Autodesk Fusion 360 part; units mm, degrees
sketch "Sketch1" plane through (0, 0, 0) normal (0, 0, 1) x (1, 0, 0)
  line L0 (-40, -75) -> (40, -75)
  line L1 (90, -25) -> (90, 25)
  line L2 (40, 75) -> (-40, 75)
  line L3 (-90, 25) -> (-90, -25)
  line L4 (-90, -75) -> (90, 75) construction
  line L5 (90, -75) -> (-90, 75) construction
  arc A0 (40, -75) -> (90, -25) centre (40, -25) ccw
  arc A1 (90, 25) -> (40, 75) centre (40, 25) ccw
  arc A2 (-90, -25) -> (-40, -75) centre (-40, -25) ccw
  arc A3 (-40, 75) -> (-90, 25) centre (-40, 25) ccw
extrude "Extrude1" add sketch "Sketch1" along normal blind 30
sketch "Sketch2" plane through (0, 0, 30) normal (0, 0, 1) x (-1, 0, 0)
  arc A0 (40, -75) -> (90, -25) centre (40, -25) ccw
  line L0 (90, -25) -> (90, 25)
  arc A1 (90, 25) -> (40, 75) centre (40, 25) ccw
  line L1 (40, 75) -> (-40, 75)
  arc A2 (-40, 75) -> (-90, 25) centre (-40, 25) ccw
  line L2 (-90, 25) -> (-90, -25)
  arc A3 (-90, -25) -> (-40, -75) centre (-40, -25) ccw
  line L3 (-40, -75) -> (40, -75)
  line L4 (35, 70) -> (-35, 70)
  line L5 (-85, 20) -> (-85, -20)
  line L6 (-35, -70) -> (35, -70)
  line L7 (85, -20) -> (85, 20)
  line L8 (85, 70) -> (-85, -70) construction
  line L9 (-85, 70) -> (85, -70) construction
  arc A4 (-35, 70) -> (-85, 20) centre (-35, 20) ccw
  arc A5 (-85, -20) -> (-35, -70) centre (-35, -20) ccw
  arc A6 (85, 20) -> (35, 70) centre (35, 20) ccw
  arc A7 (35, -70) -> (85, -20) centre (35, -20) ccw
  dimension "d9" = 140
  dimension "d10" = 170
  dimension "d11" = 50
  dimension "d12" = 50
  dimension "d13" = 50
  dimension "d14" = 50
extrude "Extrude2" cut sketch "Sketch2" against normal blind 10 contours L4 L5 L6 L7 A4 A5 A6 A7
sketch "Sketch3" plane through (0, 0, 0) normal (0, 0, -1) x (1, 0, 0)
  arc A0 (-90, -25) -> (-40, -75) centre (-40, -25) ccw
  line L0 (-40, -75) -> (40, -75)
  arc A1 (40, -75) -> (90, -25) centre (40, -25) ccw
  line L1 (90, -25) -> (90, 25)
  arc A2 (90, 25) -> (40, 75) centre (40, 25) ccw
  line L2 (40, 75) -> (-40, 75)
  arc A3 (-40, 75) -> (-90, 25) centre (-40, 25) ccw
  line L3 (-90, 25) -> (-90, -25)
  line L4 (-35, -70) -> (35, -70)
  line L5 (85, -20) -> (85, 20)
  line L6 (35, 70) -> (-35, 70)
  line L7 (-85, 20) -> (-85, -20)
  line L8 (-85, -70) -> (85, 70) construction
  line L9 (85, -70) -> (-85, 70) construction
  arc A4 (35, -70) -> (85, -20) centre (35, -20) ccw
  arc A5 (85, 20) -> (35, 70) centre (35, 20) ccw
  arc A6 (-85, -20) -> (-35, -70) centre (-35, -20) ccw
  arc A7 (-35, 70) -> (-85, 20) centre (-35, 20) ccw
  dimension "d17" = 140
  dimension "d18" = 170
  dimension "d19" = 50
  dimension "d20" = 50
  dimension "d21" = 50
  dimension "d22" = 50
extrude "Extrude3" cut sketch "Sketch3" against normal blind 10 contours L4 L5 L6 L7 A4 A5 A6 A7
sketch "Sketch4" plane through (0, 0, 10) normal (0, 0, -1) x (1, 0, 0)
  arc A0 (-35, 70) -> (-85, 20) centre (-35, 20) ccw
  line L0 (-85, 20) -> (-85, -20)
  arc A1 (-85, -20) -> (-35, -70) centre (-35, -20) ccw
  line L1 (-35, -70) -> (35, -70)
  arc A2 (35, -70) -> (85, -20) centre (35, -20) ccw
  line L2 (85, -20) -> (85, 20)
  arc A3 (85, 20) -> (35, 70) centre (35, 20) ccw
  line L3 (35, 70) -> (-35, 70)
  line L4 (90, 0) -> (45, 0)
  circle A4 centre (45, 0) radius 5.5
  dimension "d25" = 45
  dimension "d26" = 11
extrude "Extrude4" cut sketch "Sketch4" against normal blind 10 contours A4
extrude "Extrude5" add 1 faces at (-26.8129, 30.2732, 20) along direction (0, 0, 1) blind 10
extrude "Extrude6" add 1 faces at (-26.8129, 30.2732, 10) along direction (0, 0, -1) blind 10
sketch "Sketch5" plane through (0, 0, 0) normal (0, 0, -1) x (1, 0, 0)
  circle A0 centre (45, 0) radius 5.5
  arc A1 (-90, -25) -> (-40, -75) centre (-40, -25) ccw
  line L0 (-40, -75) -> (40, -75)
  arc A2 (40, -75) -> (90, -25) centre (40, -25) ccw
  line L1 (90, -25) -> (90, 25)
  arc A3 (90, 25) -> (40, 75) centre (40, 25) ccw
  line L2 (40, 75) -> (-40, 75)
  arc A4 (-40, 75) -> (-90, 25) centre (-40, 25) ccw
  line L3 (-90, 25) -> (-90, -25)
  line L4 (-75, 50) -> (-50, 50)
  line L5 (-50, 50) -> (-50, -50)
  line L6 (-50, -50) -> (-75, -50)
  line L7 (-75, -50) -> (-75, 50)
extrude "Extrude7" cut sketch "Sketch5" against normal blind 65 contours L4 L5 L6 L7
Design review of the part built by this model. Coordinates are the model's own, in mm. A direction names the side the tool comes from. Round coordinates to 2 decimals unless told otherwise and drop trailing zeros. Write each loop counter-clockwise with the first axis right and the second up, starting at its lowest first coordinate (ties: lowest second). Pieces come first, ordered by that corner, then holes. Notation, with made-up numbers: (24, 2) - (80, 2) arc R25 cw to (80, 17) - close; hole circle Ø8 at (-20.75, 83). An arc over 180 degrees is marked (long way). Use a Markdown table: item, result. Add a question column.
1. We need section D-D (y = -43). State the section outline as (x, z) points, then the cut area to 3 significant figures.
2. For faces 4 (the face through (-75, 1, 15)), 5 (the face through (-74.964, -60.742, 14.79)), list the 3-axis set-ups (+Z, -Z, +X, -X, +Y, -Y) from which the entire face can be reached by the end or side of a thin tool; tool diameter is ignored.
3. We need section B-B (z = 6.75). State the section outline as (x, y) points.
4. Wall thickness on probe 1 along X at (y, z) = (0, 7.25); probe 2 along X at (y, z) = (17.5, 28.25); probe 3 along X at (y, z) = (-2.5, 26): over which ranges is each line inside the solid? List them lowest first.
5. Clearance check with flat-ended pins moving along their axes: pin 1 (5 mm diameter, centred on y = -39, z = 18.5, fed in from -X); pin 2 (5 mm diameter, centred on x = -71.5, y = 24, fed in from +Z); pin 3 (7.5 mm diameter, centred on x = -68.5, z = 11.5, fed in from -Y); pin 4 (4 mm diameter, centred on x = -40.5, z = 27, fed in from -Y). State where each tip first meets the part, or that it passes through.
6. Mouldability with a two-part tool opening along X and no side actions: class faces 1 (the face through (39.505, -0.242, 14.79)), 2 (the face through (90, 0, 15)), 3 (the face through (-1, -75, 15)) as +X half, -X half, draft (parallel to the pull), parting line (faces both ways), or undercut.
7. We need section A-A (y = 0). State the section outline as (x, z) points, then the cut area to 3 significant figures.
8. We need section C-C (x = 45). State the section outline as (y, z) points, then the cut area to 3 significant figures.
Output:
| question | item | result |
|---|---|---|
| 1 | outline | (-86.65, 0) - (-75, 0) - (-75, 30) - (-86.65, 30) - close; (-50, 0) - (86.65, 0) - (86.65, 30) - (-50, 30) - close |
| 1 | area | 4,450 mm2 |
| 2 | face 4 | +Z, -Z |
| 2 | face 5 | +Z, -Z, -X, -Y |
| 3 | outline | (-90, -25) arc R50 ccw to (-40, -75) - (40, -75) arc R50 ccw to (90, -25) - (90, 25) arc R50 ccw to (40, 75) - (-40, 75) arc R50 ccw to (-90, 25) - close; hole (-75, -50) - (-50, -50) - (-50, 50) - (-75, 50) - close; hole circle Ø11 at (45, 0) |
| 4 | probe 1 | x = -90 to -75, -50 to 39.5, 50.5 to 90 |
| 4 | probe 2 | x = -90 to -75, -50 to 90 |
| 4 | probe 3 | x = -90 to -75, -50 to 40.1, 49.9 to 90 |
| 5 | pin 1 | stops at x = -88.66 |
| 5 | pin 2 | passes through |
| 5 | pin 3 | stops at y = -68.44 |
| 5 | pin 4 | stops at y = -75 |
| 6 | face 1 | undercut |
| 6 | face 2 | +X half |
| 6 | face 3 | draft |
| 7 | outline | (-90, 0) - (-75, 0) - (-75, 30) - (-90, 30) - close; (-50, 0) - (39.5, 0) - (39.5, 30) - (-50, 30) - close; (50.5, 0) - (90, 0) - (90, 30) - (50.5, 30) - close |
| 7 | area | 4,320 mm2 |
| 8 | outline | (-74.75, 0) - (-5.5, 0) - (-5.5, 30) - (-74.75, 30) - close; (5.5, 0) - (74.75, 0) - (74.75, 30) - (5.5, 30) - close |
| 8 | area | 4,150 mm2 |
